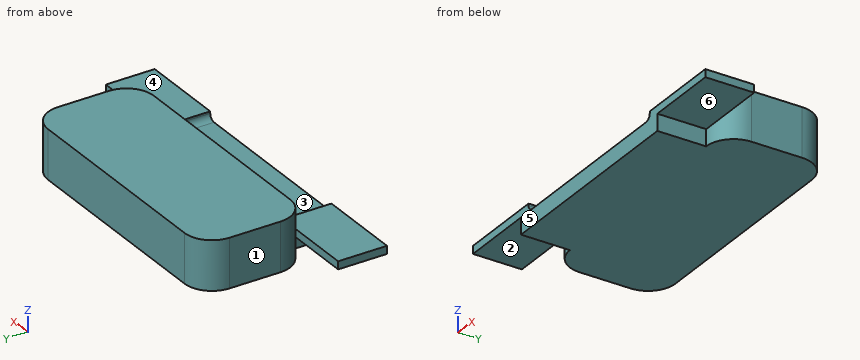
```python
from build123d import *

# Parameters (mm, degrees)
F1_DEPTH = 12.5
F5_DEPTH = 25


# Not quite as in the source:
# - the program builds the solid bodies; features that only make, move or delete a surface that nothing else refers to are left out


with BuildPart() as f1:
    # F0 (on Top) → F1 (new body, symmetric)
    with BuildSketch(Plane.XY):
        with BuildLine():
            Line((-122, 0), (-14, 0))
            ThreePointArc((-14, 0), (-4.1005050634, 4.1005050634), (0, 14))
            Line((0, 14), (0, 40))
            ThreePointArc((0, 40), (-4.1005050634, 49.8994949366), (-14, 54))
            Line((-14, 54), (-122, 54))
            ThreePointArc((-122, 54), (-131.8994949366, 49.8994949366), (-136, 40))
            Line((-136, 40), (-136, 14))
            ThreePointArc((-136, 14), (-131.8994949366, 4.1005050634), (-122, 0))
        make_face()
    extrude(amount=F1_DEPTH, both=True)

    # F4 (on face) → F5 (join)
    with BuildSketch(Plane.XZ):
        with BuildLine():
            Line((-122, -4), (-122, -12.5))
            Line((-122, -12.5), (-14, -12.5))
            Line((-14, -12.5), (-14, -4))
            Line((-14, -4), (24, -4))
            Line((24, -4), (24, 0))
            Line((24, 0), (-20, 0))
            Line((-20, 0), (-20, -1))
            ThreePointArc((-20, -1), (-20.8786796564, -3.1213203436), (-23, -4))
            Line((-23, -4), (-113, -4))
            ThreePointArc((-113, -4), (-115.1213203436, -3.1213203436), (-116, -1))
            Line((-116, -1), (-116, 0))
            Line((-116, 0), (-160, 0))
            Line((-160, 0), (-160, -4))
            Line((-160, -4), (-122, -4))
        make_face()
    extrude(amount=F5_DEPTH)


solid = f1.part
```
The model under review builds one solid part; all positions refer to its coordinate system, in mm. Face numbers are marked on the shaded views. A direction names the side the tool comes from. Round coordinates to 2 decimals unless told otherwise and drop trailing zeros. Loops run counter-clockwise (first coordinate to the right, second up) from the corner with the lowest first, then second, coordinate; pieces in that order, holes last.
1) Consider section C-C on z = -6. State the section outline as (x, y) points, then the cut area to 3 significant figures.
Values follow:
outline: (-136, 14) arc R14 ccw to (-122, 0) - (-122, -25) - (-14, -25) - (-14, 0) arc R14 ccw to (0, 14) - (0, 40) arc R14 ccw to (-14, 54) - (-122, 54) arc R14 ccw to (-136, 40) - close
area: 9,880 mm2
2) Consider section B-B on y = -10.5. State the section outline as (x, z) points.
Values follow:
outline: (-160, -4) - (-122, -4) - (-122, -12.5) - (-14, -12.5) - (-14, -4) - (24, -4) - (24, 0) - (-20, 0) - (-20, -1) arc R3 cw to (-23, -4) - (-113, -4) arc R3 cw to (-116, -1) - (-116, 0) - (-160, 0) - close
3) Wall thickness on line 1 along X through (y, z) = (-1, -0.75); line 2 along X through (y, z) = (27.5, -4.25); line 3 along Z through (x, y) = (9, -11.5): over which ranges is each line inside the solid? List them lowest first.
Values follow:
line 1: x = -160 to -116, -20 to 24
line 2: x = -136 to 0
line 3: z = -4 to 0
4) Consider section A-A on x = -128.5. State the section outline as (y, z) points.
Values follow:
outline: (-25, -4) - (0, -4) - (0, 0) - (-25, 0) - close; (1.6, -12.5) - (52.4, -12.5) - (52.4, 12.5) - (1.6, 12.5) - close
5) Clearance check with flat-ended pins moving along their axes: P1, Ø7.5, axis at x = 14, y = -8, coming from the -Z side; P2, Ø7, axis at y = -12.5, z = -9.5, coming from the +X side; P3, Ø10, axis at y = 18.5, z = 9.5, coming from the +X side; P4, Ø4, axis at x = -138.5, y = 39.5, coming from the +Z side. State where each tip first meets the part, or that it passes through.
Values follow:
P1: stops at z = -4
P2: stops at x = -14
P3: stops at x = 0
P4: passes through
6) The part is to be moulded in two halves that separate along X. For the marked faces 1, 2 and 3, say which applies: pulls with the +X half, pulls with the -X half, needs draft (parallel to the pull), parting line crosses it, or undercut.
Values follow:
face 1: pulls with the -X half
face 2: needs draft
face 3: undercut
7) Tool access review of the marked faces 4, 5 and 6: name each direction out of +Z, -Z, +X, -X, +Y, -Y from which nothing blocks a thin tool from reaching the whole face with its end or side.
Values follow:
face 4: +Z, +X, -X, -Y
face 5: +Z, -Z, +X, -X, -Y
face 6: -Z, +X, -Y
8) Consider section D-D on x = -36.5. State the section outline as (y, z) points, then the cut area to 3 significant figures.
Values follow:
outline: (-25, -12.5) - (54, -12.5) - (54, 12.5) - (0, 12.5) - (0, -4) - (-25, -4) - close
area: 1,560 mm2
